Could you check a few things on this model? Use its own coordinates, in mm. Coordinates: 2 decimals unless noted, no trailing zeros. Loops run counter-clockwise (first coordinate to the right, second up) from the corner with the lowest first, then second, coordinate; pieces in that order, holes last. Notation, with made-up numbers: (43, 21) - (50, 21) arc R30 cw to (50, 52) - close; hole circle Ø4 at (53.25, -39.5). An arc over 180 degrees is marked (long way). One line per item, written item: value. Start each with the question number.
(1) If we section it at C-C on x = 195: Write out the boundary of the cut face in (y, z).
(2) If we section it at D-D on x = 7.5: Write out the boundary of the cut face in (y, z), then the cut area to 3 significant figures.
(3) I'm going to push flat-ended pins straight in: P1, Ø7.5, axis at x = 88.5, z = 10.5, coming from the +Y side; P2, Ø5, axis at x = 138.5, z = 2, coming from the -Y side. Where does each tip first touch, or does it pass through?
(4) If we section it at A-A on y = -60: Write out the boundary of the cut face in (x, z).
(5) If we section it at B-B on z = 7.5: Write out the boundary of the cut face in (x, y), then the cut area to 3 significant figures.
(6) If I drill on line 1 along Y through (x, z) = (195, 6); line 2 along Y through (x, z) = (23, 10.5); line 3 along Y through (x, z) = (191, 11.5), over which ranges is the centre line in solid material (lowest first)? Write a range as from..to.
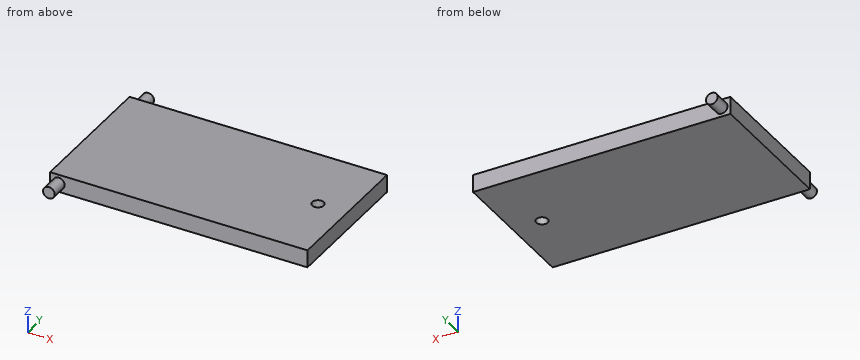
```python
from build123d import *

# Parameters (mm, degrees)
SKETCH1_W                = 220
SKETCH1_H                = 120
BOSS_EXTRUDE1_DEPTH      = 15
BOSS_EXTRUDE2_DEPTH      = 15
BOSS_EXTRUDE2_DEPTH_BACK = 135
SKETCH2_R                = 5
SKETCH3_R                = 5
CUT_EXTRUDE1_DEPTH       = 25


with BuildPart() as part:
    # Sketch1 → Boss-Extrude1 (new body)
    with BuildSketch(Plane.XY):
        with Locations((110, -60)):
            Rectangle(SKETCH1_W, SKETCH1_H)
    extrude(amount=BOSS_EXTRUDE1_DEPTH)

    # Sketch2 → Boss-Extrude2 (add, two sides: drawn at the far end of the back side and taken through both)
    with BuildSketch(Plane(origin=(0, 0, 0), x_dir=(1, 0, 0), z_dir=(0, 1, 0)).offset(-BOSS_EXTRUDE2_DEPTH_BACK)):
        with Locations(Location((7.5, -7.5, 0), (0, 0, 270))):
            Circle(SKETCH2_R)
    extrude(amount=BOSS_EXTRUDE2_DEPTH + BOSS_EXTRUDE2_DEPTH_BACK)

    # Sketch3 → Cut-Extrude1 (cut)
    with BuildSketch(Plane.XY.offset(15)):
        with Locations((195, -60)):
            Circle(SKETCH3_R)
    extrude(amount=-CUT_EXTRUDE1_DEPTH, mode=Mode.SUBTRACT)


solid = part.part
```
Values:
1. outline: (-120, 0) - (-65, 0) - (-65, 15) - (-120, 15) - close; (-55, 0) - (0, 0) - (0, 15) - (-55, 15) - close
2. outline: (-135, 2.5) - (-120, 2.5) - (-120, 0) - (0, 0) - (0, 2.5) - (15, 2.5) - (15, 12.5) - (0, 12.5) - (0, 15) - (-120, 15) - (-120, 12.5) - (-135, 12.5) - close
2. area: 2,100 mm2
3. P1: stops at y = 0
3. P2: stops at y = -120
4. outline: (0, 0) - (190, 0) - (190, 15) - (0, 15) - close; (200, 0) - (220, 0) - (220, 15) - (200, 15) - close
5. outline: (0, -120) - (2.5, -120) - (2.5, -135) - (12.5, -135) - (12.5, -120) - (220, -120) - (220, 0) - (12.5, 0) - (12.5, 15) - (2.5, 15) - (2.5, 0) - (0, 0) - close; hole circle Ø10 at (195, -60)
5. area: 26,600 mm2
6. line 1: y = -120..-65, -55..0
6. line 2: y = -120..0
6. line 3: y = -120..-63, -57..0
